Can you work these out from the model? Positions are in its coordinate system, mm. Face numbers are marked on the shaded views. A direction names the side the tool comes from. Coordinates: 2 decimals unless noted, no trailing zeros. Write each loop counter-clockwise with the first axis right and the second up, starting at its lowest first coordinate (ties: lowest second). Pieces come first, ordered by that corner, then holes. Notation, with made-up numbers: M 44.25,-1 L 57.25,-1 A22 ccw 57.25,9 Z; hole C 39.25,41 d6. An arc over 180 degrees is marked long. Answer as a JSON object with one key per item and string values. Group by question number.
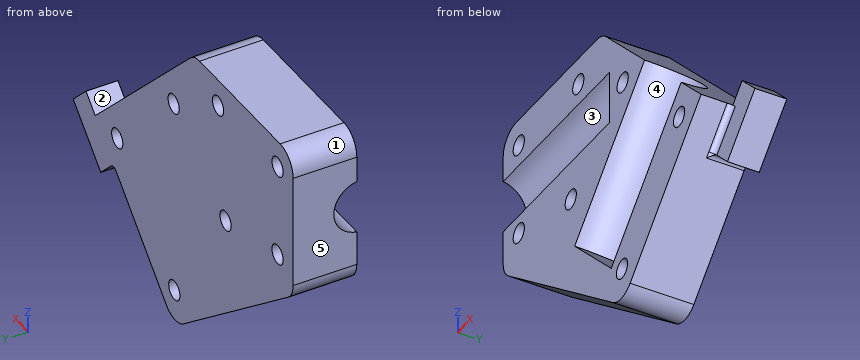
from build123d import *

# Parameters (mm, degrees)
EXTRUDE_1_DEPTH        = 14
EXTRUDE_2_DEPTH        = 7
CUT_EXTRUDE_1_DEPTH    = 38.1
CUT_EXTRUDE_2_DEPTH    = 41.028932188
HOLE_WIZARD_M4_1_D     = 4.318
HOLE_WIZARD_M4_1_DEPTH = 14
FILLET_1_R             = 5
FILLET_3_R             = 1.27
FILLET_4_R             = 1.27


with BuildPart() as part:
    # 草图1 → 凸台-拉伸1 (new body)
    with BuildSketch(Plane.XZ.offset(-1)):
        Polygon((4.743453393, -52.27499012), (35.219755662, -21.79868785), (-2.928932188, 16.35), (-41.028932188, 16.35), (-41.028932188, -16.35), align=None)
    extrude(amount=-EXTRUDE_1_DEPTH)

    # 草图2 → 凸台-拉伸2 (add)
    with BuildSketch(Plane(origin=(0, 15, 0), x_dir=(1, 0, 0), z_dir=(0, 1, 0))):
        Polygon((35.219755662, 21.79868785), (38.755289568, 18.263153944), (43.705037037, 23.212901413), (33.098435319, 33.819503131), (28.14868785, 28.869755662), align=None)
    extrude(amount=-EXTRUDE_2_DEPTH)

    # 草图3 → 切除-拉伸1 (cut)
    with BuildSketch(Plane(origin=(6.710533906, 0, 6.710533906), x_dir=(0.707106781, 0, -0.707106781), z_dir=(0.707106781, 0, 0.707106781))):
        with BuildLine():
            Line((9.538251542, 1), (29.445830798, 1))
            ThreePointArc((29.445830798, 1), (19.49204117, 10.039754177), (9.538251542, 1))
        make_face()
    extrude(amount=-CUT_EXTRUDE_1_DEPTH, mode=Mode.SUBTRACT)

    # 草图4 → 切除-拉伸2 (cut)
    with BuildSketch(Plane.ZY.offset(41.028932188)):
        with BuildLine():
            Line((-6.270765504, 1), (5.579500015, 1))
            ThreePointArc((5.579500015, 1), (-0.345632744, 6.05511811), (-6.270765504, 1))
        make_face()
    extrude(amount=-CUT_EXTRUDE_2_DEPTH, mode=Mode.SUBTRACT)

    # M4 间隙孔1
    with Locations(Plane(origin=(0, 15, 0), x_dir=(1, 0, 0), z_dir=(0, 1, 0))):
        with Locations((-35.028932188, -10.35), (5, 0), (-15, 15), (-12.103043109, -10.35), (-35.028932188, 10.35), (4.743453393, 43.789708745), (26.734474288, 21.79868785)):
            Hole(HOLE_WIZARD_M4_1_D / 2, depth=HOLE_WIZARD_M4_1_DEPTH)

    # 圆角1
    fillet_1_edges = [part.edges().sort_by_distance(p)[0] for p in [
        (-41.028932188, 8, -16.35),
        (-41.028932188, 8, 16.35),
        (-2.928932188, 8, 16.35),
        (4.743453393, 8, -52.27499012),
    ]]
    fillet(fillet_1_edges, radius=FILLET_1_R)

    # 圆角3
    fillet_3_edges = [part.edges().sort_by_distance(p)[0] for p in [
        (28.14868785, 11.5, -28.869755662),
    ]]
    fillet(fillet_3_edges, radius=FILLET_3_R)

    # 圆角4
    fillet_4_edges = [part.edges().sort_by_distance(p)[0] for p in [
        (31.684221756, 8, -25.334221756),
    ]]
    fillet(fillet_4_edges, radius=FILLET_4_R)


solid = part.part
Q1. If we section it at A-A on z = 10.35: List the corners of the cut face in (x, y) for me, and give its area (3 significant figures).
Q2. On a 3-axis mill with a long thin cutter (end or side, diameter ignored), from which of +Z, -Z, +X, -X, +Y, -Y can I reach the whole of each face in a straight line? I mean the marked faces 1 and 2. Say none if no direction works.
Q3. Will these pins go through, and if not, where does the flat tip stop? pin 1 (5 mm diameter, centred on x = -24, y = 13.5, fed in from -Z); pin 2 (6 mm diameter, centred on x = -22.5, y = 8.5, fed in from -Z); pin 3 (5.5 mm diameter, centred on x = 5, z = 0, fed in from -Y); pin 4 (3 mm diameter, centred on x = 35, y = 13.5, fed in from +Z).
Q4. If we section it at D-D on y = 11: List the corners of the cut face in (x, z) for me.
Q5. We'd pull the mould along X, two halves only. Please class the marked faces 3, 4 and 5: pulls with the +X half, pulls with the -X half, needs draft (parallel to the pull), parting line crosses it, or undercut.
Q6. If we section it at C-C on x = 5: Give the number of separate pieces and of enclosed holes in the cut face, and give its area (3 significant figures).
Q7. Please list where these lines run through material, in increasing order: L1, parallel to Z at x = -33.5, y = 8.5; L2, parallel to X at y = 8, z = 1; L3, parallel to X at y = 7, z = 10.35.
Q8. If we section it at B-B on y = 4: List the corners of the cut face in (x, z) for me, and give its area (3 significant figures).
Reply:
{
 "1": {"outline": "M -41.03,1 L -37.19,1 L -37.19,15 L -41.03,15 Z; M -32.87,1 L -14.26,1 L -14.26,15 L -32.87,15 Z; M -9.94,1 L 3.07,1 L 3.07,15 L -9.94,15 Z", "area": "496 mm^2"},
 "2": {"face 1": "+Z, -X, +Y, -Y", "face 2": "+Z, +Y, -Y"},
 "3": {"pin 1": "z = -31.68", "pin 2": "z = -33.25", "pin 3": "y = 1", "pin 4": "z = -20.08"},
 "4": {"outline": "M -41.03,-13.92 A5 ccw -39.12,-17.85 L 1.26,-49.54 A5 ccw 7.88,-49.14 L 27.25,-29.77 A1.27 cw 29.05,-29.77 L 33.1,-33.82 L 43.71,-23.21 L 38.76,-18.26 L 35.22,-21.8 L -1.46,14.89 A5 ccw -5,16.35 L -36.03,16.35 A5 ccw -41.03,11.35 Z; hole C -35.03,-10.35 d4.32; hole C -35.03,10.35 d4.32; hole C -15,-15 d4.32; hole C -12.1,10.35 d4.32; hole C 4.74,-43.79 d4.32; hole C 5,0 d4.32; hole C 26.73,-21.8 d4.32"},
 "5": {"face 3": "needs draft", "face 4": "undercut", "face 5": "pulls with the -X half"},
 "6": {"separate pieces": "3", "enclosed holes": "0", "area": "510 mm^2"},
 "7": {"L1": "-22.26 to -11.87, -8.83 to 8.83, 11.87 to 16.35", "L2": "-41.03 to 3.09, 6.91 to 12.42", "L3": "-41.03 to -37.19, -32.87 to -14.26, -9.94 to 3.07"},
 "8": {"outline": "M -41.03,-13.92 A5 ccw -39.12,-17.85 L 1.26,-49.54 A5 ccw 7.88,-49.14 L 35.22,-21.8 L 26.99,-13.57 L 0.05,-40.51 L -12.94,-27.52 L 14,-0.58 L -1.46,14.89 A5 ccw -5,16.35 L -36.03,16.35 A5 ccw -41.03,11.35 L -41.03,4.18 L 0,4.18 L 0,-4.87 L -41.03,-4.87 Z; hole C -35.03,-10.35 d4.32; hole C -35.03,10.35 d4.32; hole C -15,-15 d4.32; hole C -12.1,10.35 d4.32; hole C 4.74,-43.79 d4.32; hole C 5,0 d4.32; hole C 26.73,-21.8 d4.32", "area": "2,030 mm^2"}
}
